```python
from build123d import *

# Parameters (mm, degrees)
SKETCH_1_R          = 6.5
SKETCH_1_R_2        = 2
EXTRUDE_1_DEPTH     = 6
SKETCH_2_R          = 5
SKETCH_2_R_2        = 3
CUT_EXTRUDE_1_DEPTH = 1
CUT_EXTRUDE_START   = -1
SKETCH_3_R          = 5
SKETCH_3_R_2        = 3
CUT_EXTRUDE_2_DEPTH = 1
SKETCH_4_W          = 1
SKETCH_4_H          = 2
FILLET_1_R          = 1
FILLET_2_R          = 1.5


with BuildPart() as part:
    # 草图1 → 凸台-拉伸1 (new body)
    with BuildSketch(Plane(origin=(0, 0, 0), x_dir=(1, 0, 0), z_dir=(0, 1, 0))):
        with Locations(Location((0, 0, 0), (0, 0, 270))):
            Circle(SKETCH_1_R)
        with Locations(Location((0, 0, 0), (0, 0, 270))):
            Circle(SKETCH_1_R_2, mode=Mode.SUBTRACT)
    extrude(amount=EXTRUDE_1_DEPTH)

    # 草图2 → 切除-拉伸1 (cut)
    with BuildSketch(Plane(origin=(0, 6, 0), x_dir=(1, 0, 0), z_dir=(0, 1, 0))):
        with Locations(Location((0, 0, 0), (0, 0, 270))):
            Circle(SKETCH_2_R)
        with Locations(Location((0, 0, 0), (0, 0, 270))):
            Circle(SKETCH_2_R_2, mode=Mode.SUBTRACT)
    extrude(amount=-CUT_EXTRUDE_1_DEPTH, mode=Mode.SUBTRACT)

    # 草图3 → 切除-拉伸2 (cut)
    with BuildSketch(Plane(origin=(0, 0, 0), x_dir=(-1, 0, 0), z_dir=(0, -1, 0)).offset(CUT_EXTRUDE_START)):
        with Locations(Location((0, 0, 0), (0, 0, 270))):
            Circle(SKETCH_3_R)
        with Locations(Location((0, 0, 0), (0, 0, 270))):
            Circle(SKETCH_3_R_2, mode=Mode.SUBTRACT)
    extrude(amount=CUT_EXTRUDE_2_DEPTH, mode=Mode.SUBTRACT)

    # 草图4 → 切除-旋转1 (revolve, cut)
    with BuildSketch(Plane.XY, mode=Mode.PRIVATE) as cut_revolve_1_sk:
        with Locations((6, 3)):
            Rectangle(SKETCH_4_W, SKETCH_4_H)
    revolve(cut_revolve_1_sk.sketch.rotate(Axis((0, 0, 0), (0, 1, 0)), 90), axis=Axis((0, 0, 0), (0, 1, 0)), mode=Mode.SUBTRACT)

    # 圆角1
    fillet_1_edges = [part.edges().sort_by_distance(p)[0] for p in [
        (0, 2, 5.5),
        (0, 4, 5.5),
    ]]
    fillet(fillet_1_edges, radius=FILLET_1_R - 0.0001)  # a hair under: the kernel refuses the full size

    # 圆角2
    fillet_2_edges = [part.edges().sort_by_distance(p)[0] for p in [
        (0, 4, -6.5),
        (0, 2, -6.5),
    ]]
    fillet(fillet_2_edges, radius=FILLET_2_R)


solid = part.part
```
Model file for the job. Use its own axes, mm. A direction names the side the tool comes from. Round coordinates to 2 decimals unless told otherwise and drop trailing zeros. Put each result on its own line as item: value. Start each with the question number.
Item 1: 3-axis set-ups, long thin cutter, end or side, ignore diameter. For faces 1 (the face through (-3.955, 0.493, -5.158)), 2 (the face through (-3.3, 5, -0.1)), 3 (the face through (-0.9, 0.51, 2.86)): which of +Z, -Z, +X, -X, +Y, -Y reach the whole face in a straight line?
Item 2: Drill centre lines: line 1 along X through (y, z) = (5.65, 0); line 2 along Y through (x, z) = (-1.25, 3); line 3 along Z through (x, y) = (1, 5.75). Where is each one in solid material? Low to high.
Item 3: Drop flat-ended pins along their axis: P1, Ø1, axis at y = 4, z = 3, coming from the -X side; P2, Ø1, axis at x = -3, z = -3, coming from the -Y side. Give the stop position or say it passes through.
Answer block:
1. face 1: +Y, -Y
1. face 2: +Y
1. face 3: -Y
2. line 1: -6.5 to -5, -3 to -2, 2 to 3, 5 to 6.5
2. line 2: 1 to 5
2. line 3: -6.42 to -4.9, -2.83 to -1.73, 1.73 to 2.83, 4.9 to 6.42
3. P1: x = -5.78
3. P2: y = 1
